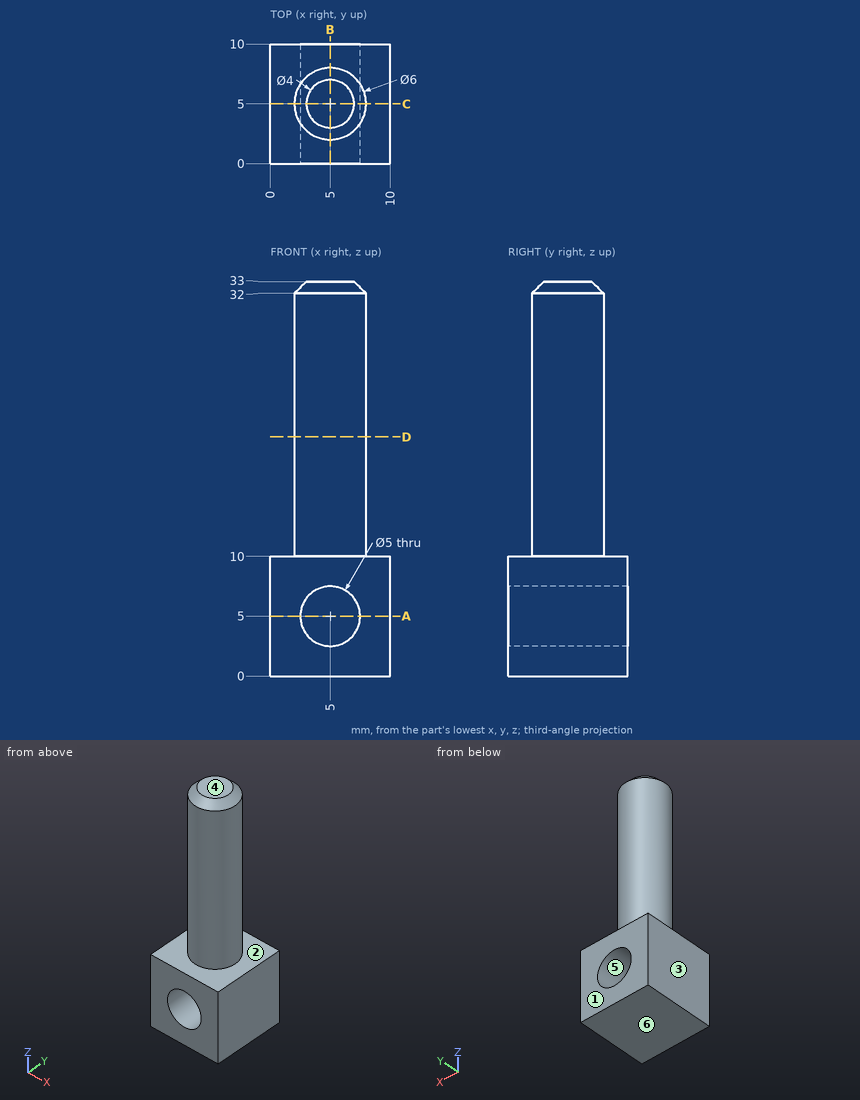
The drawing under review shows one solid part. Ordinate dimensions are in mm from its lowest x, y, z. A direction names the side the tool comes from. Round coordinates to 2 decimals unless told otherwise and drop trailing zeros. Loops run counter-clockwise (first coordinate to the right, second up) from the corner with the lowest first, then second, coordinate; pieces in that order, holes last. Notation, with made-up numbers: (5.25, -38.75) -> (12.25, -38.75) arc R15 ccw to (12.25, -14.75) -> close; hole circle Ø5 at (33.5, -4). An arc over 180 degrees is marked (long way). Answer in a Markdown table with one row per item.
1) For pin 1 Ø1.5 at (x, y) = (9, 8) entering from +Z; pin 2 Ø1 at (x, y) = (8, 4.5) entering from +Z; pin 3 Ø3 at (x, z) = (7.5, 27) entering from -Y, all flat-tipped, find the tip position at first contact; note any pin that passes through.
Taken from the geometry:
| item | result |
|---|---|
| pin 1 | stops at z = 10 |
| pin 2 | stops at z = 32.46 |
| pin 3 | stops at y = 2.17 |
2) Consider section D-D, the plane z = 20. Write out the cut boundary in (x, y).
Taken from the geometry:
| item | result |
|---|---|
| outline | circle Ø6 at (5, 5) |
3) Consider section A-A, the plane z = 5. Write out the cut boundary in (x, y), plus the area to 3 significant figures.
Taken from the geometry:
| item | result |
|---|---|
| outline | (0, 0) -> (2.5, 0) -> (2.5, 10) -> (0, 10) -> close; (7.5, 0) -> (10, 0) -> (10, 10) -> (7.5, 10) -> close |
| area | 50.0 mm² |
4) Wall thickness on line 1 along Z through (x, y) = (5, 7); line 2 along Z through (x, y) = (3.5, 9); line 3 along X through (y, z) = (9.5, 3): over which ranges is each line inside the solid? List them lowest first.
Taken from the geometry:
| item | result |
|---|---|
| line 1 | z = 0 to 2.5, 7.5 to 33 |
| line 2 | z = 0 to 3, 7 to 10 |
| line 3 | x = 0 to 3.5, 6.5 to 10 |
5) Tool access review of the marked faces 1 and 2: name each direction out of +Z, -Z, +X, -X, +Y, -Y from which nothing blocks a thin tool from reaching the whole face with its end or side.
Taken from the geometry:
| item | result |
|---|---|
| face 1 | +Z, -Z, +X, -X, +Y |
| face 2 | +Z |
6) Draft analysis for pull direction Z (two halves, no side actions). For the marked faces 3, 4, 5 and 6, state which applies: pulls with the +Z half, pulls with the -Z half, needs draft (parallel to the pull), parting line crosses it, or undercut.
Taken from the geometry:
| item | result |
|---|---|
| face 3 | needs draft |
| face 4 | pulls with the +Z half |
| face 5 | undercut |
| face 6 | pulls with the -Z half |
7) Consider section B-B, the plane x = 5. Write out the cut boundary in (y, z), plus the area to 3 significant figures.
Taken from the geometry:
| item | result |
|---|---|
| outline | (0, 0) -> (10, 0) -> (10, 2.5) -> (0, 2.5) -> close; (0, 7.5) -> (10, 7.5) -> (10, 10) -> (8, 10) -> (8, 32) -> (7, 33) -> (3, 33) -> (2, 32) -> (2, 10) -> (0, 10) -> close |
| area | 187 mm² |
8) Consider section C-C, the plane y = 5. Write out the cut boundary in (x, z).
Taken from the geometry:
| item | result |
|---|---|
| outline | (0, 0) -> (10, 0) -> (10, 10) -> (8, 10) -> (8, 32) -> (7, 33) -> (3, 33) -> (2, 32) -> (2, 10) -> (0, 10) -> close; hole circle Ø5 at (5, 5) |
